Geometry: final body of the model. Coordinates: model frame, mm. Round coordinates to 2 decimals unless told otherwise and drop trailing zeros. Order: outer loops, then holes, each group sorted by start corner. A loop starts at its lowest first (then second) coordinate and runs counter-clockwise, first axis right, second up. Notation, with made-up numbers: (-11, 84.5) -> (48, 84.5) arc R16 ccw to (48, 102.5) -> close; hole circle Ø10 at (56.25, 38). An arc over 180 degrees is marked (long way). Put each result on its own line as item: value.
```python
from build123d import *

# Parameters (mm, degrees)
SKETCH1_R           = 1.45
BOSS_EXTRUDE1_DEPTH = 3
FILLET1_R           = 1.5


with BuildPart() as part:
    # Sketch1 → Boss-Extrude1 (new body)
    with BuildSketch(Plane.XY):
        Polygon((-20, -20), (-5, -20), (30, -55), (30, -70), (50, -70), (50, -50), (0, 0), (0, 20), (-20, 20), (-20, 0), align=None)
        with Locations((-10, -16)):
            Circle(SKETCH1_R, mode=Mode.SUBTRACT)
        with Locations((-10, -4)):
            Circle(SKETCH1_R, mode=Mode.SUBTRACT)
        with Locations((40, -52.5)):
            Circle(SKETCH1_R, mode=Mode.SUBTRACT)
        with Locations((40, -62.5)):
            Circle(SKETCH1_R, mode=Mode.SUBTRACT)
        with Locations((-10, 13)):
            Circle(SKETCH1_R, mode=Mode.SUBTRACT)
    extrude(amount=BOSS_EXTRUDE1_DEPTH)

    # Fillet1
    fillet1_edges = [part.edges().sort_by_distance(p)[0] for p in [
        (-20, 20, 1.5),
        (0, 20, 1.5),
        (0, 0, 1.5),
        (50, -50, 1.5),
        (50, -70, 1.5),
        (30, -70, 1.5),
        (30, -55, 1.5),
        (-5, -20, 1.5),
        (-20, -20, 1.5),
    ]]
    fillet(fillet1_edges, radius=FILLET1_R)


solid = part.part
```
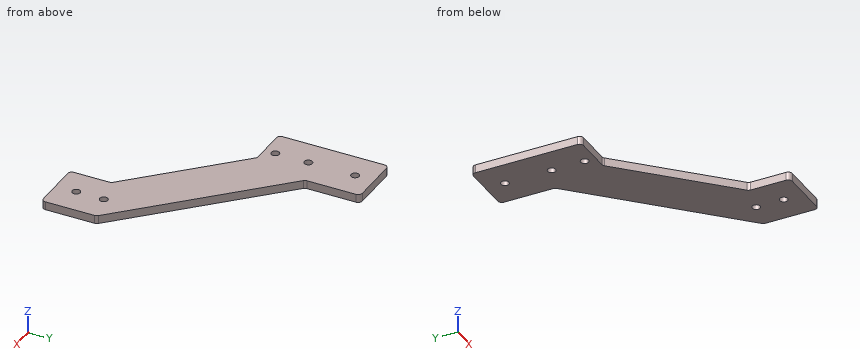
1. Cut plane C-C on x = -10. Return loops of the section in (y, z).
Ans:
outline: (-20, 0) -> (-17.45, 0) -> (-17.45, 3) -> (-20, 3) -> close; (-14.55, 0) -> (-5.45, 0) -> (-5.45, 3) -> (-14.55, 3) -> close; (-2.55, 0) -> (11.55, 0) -> (11.55, 3) -> (-2.55, 3) -> close; (14.45, 0) -> (20, 0) -> (20, 3) -> (14.45, 3) -> close
2. Cut plane A-A on y = -4. Return loops of the section in (x, z), and give its area (3 significant figures).
Ans:
outline: (-20, 0) -> (-11.45, 0) -> (-11.45, 3) -> (-20, 3) -> close; (-8.55, 0) -> (4, 0) -> (4, 3) -> (-8.55, 3) -> close
area: 63.3 mm²
3. Contact query for flat-ended pins moving along their axis: P1, Ø1.5, axis at y = 13.5, z = 2, coming from the +X side; P2, Ø1, axis at y = -20.5, z = 2, coming from the +X side. Output: stop coordinate, or through.
Ans:
P1: x = 0
P2: x = 21
4. Cut plane D-D on z = 1.75. Return loops of the section in (x, y), and give its area (3 significant figures).
Ans:
outline: (-20, -18.5) arc R1.5 ccw to (-18.5, -20) -> (-5.62, -20) arc R1.5 cw to (-4.56, -20.44) -> (29.56, -54.56) arc R1.5 cw to (30, -55.62) -> (30, -68.5) arc R1.5 ccw to (31.5, -70) -> (48.5, -70) arc R1.5 ccw to (50, -68.5) -> (50, -50.62) arc R1.5 ccw to (49.56, -49.56) -> (0.44, -0.44) arc R1.5 cw to (0, 0.62) -> (0, 18.5) arc R1.5 ccw to (-1.5, 20) -> (-18.5, 20) arc R1.5 ccw to (-20, 18.5) -> close; hole circle Ø2.9 at (-10, -16); hole circle Ø2.9 at (-10, -4); hole circle Ø2.9 at (-10, 13); hole circle Ø2.9 at (40, -62.5); hole circle Ø2.9 at (40, -52.5)
area: 2,130 mm²
5. Material intervals for probe 1 along Y at (x, z) = (-10, 0.8); probe 2 along Y at (x, z) = (40, 1.9); probe 3 along X at (y, z) = (-58.5, 0.1), sorted ascending.
Ans:
probe 1: -20 to -17.45, -14.55 to -5.45, -2.55 to 11.55, 14.45 to 20
probe 2: -70 to -63.95, -61.05 to -53.95, -51.05 to -40
probe 3: 30 to 50
6. Cut plane B-B on x = 40. Return loops of the section in (y, z), and give its area (3 significant figures).
Ans:
outline: (-70, 0) -> (-63.95, 0) -> (-63.95, 3) -> (-70, 3) -> close; (-61.05, 0) -> (-53.95, 0) -> (-53.95, 3) -> (-61.05, 3) -> close; (-51.05, 0) -> (-40, 0) -> (-40, 3) -> (-51.05, 3) -> close
area: 72.6 mm²
